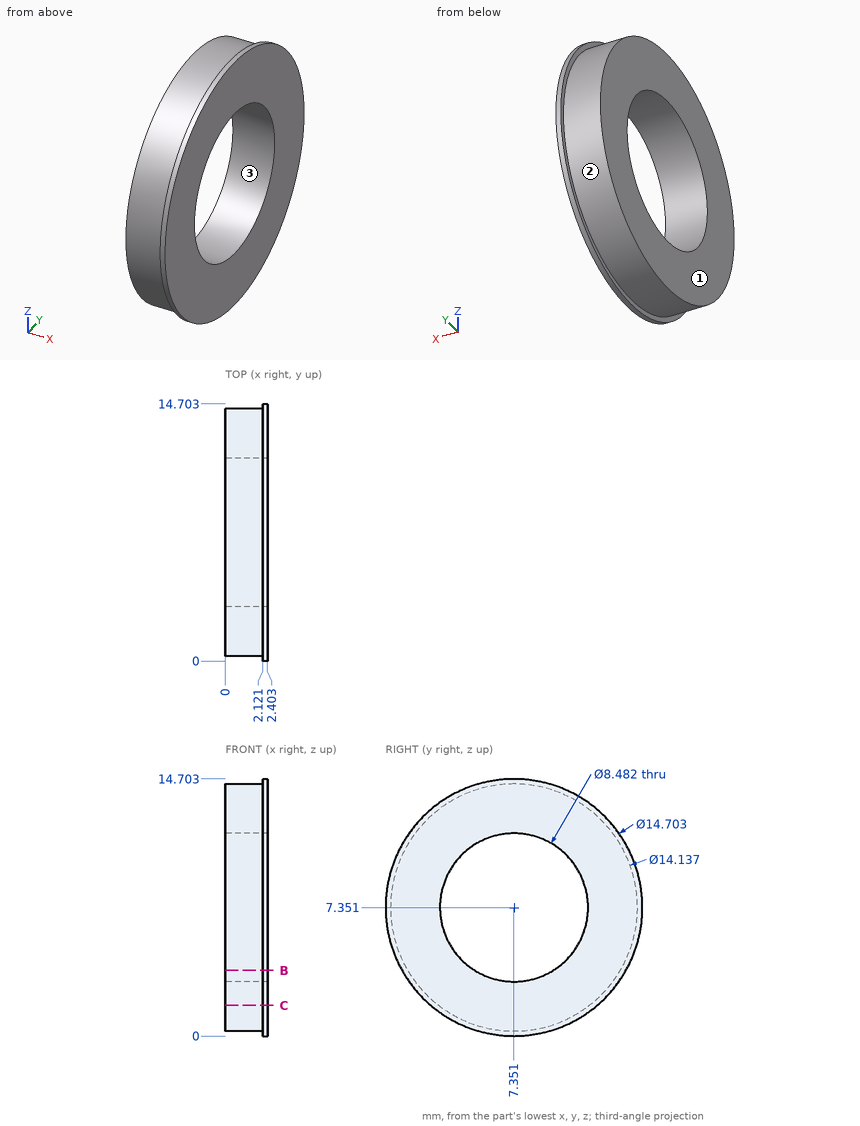
Input: dimensioned drawing with shaded views. Units: mm. Origin: part minimum x, y, z. Round coordinates to 2 decimals unless told otherwise and drop trailing zeros. Loops run counter-clockwise (first coordinate to the right, second up) from the corner with the lowest first, then second, coordinate; pieces in that order, holes last. Notation, with made-up numbers: (77, -20) -> (82, -20) arc R32 ccw to (82, 12) -> close; hole circle Ø11 at (-22.75, 70.25). An arc over 180 degrees is marked (long way). Answer as a JSON object with one key per item and string values. Group by question number.
1) Ray query, L1, parallel to Y at x = 2, z = 7.25; L2, parallel to Y at x = 1.5, z = 4.5 (1 decimal); L3, parallel to Z at x = 1.1, y = 4.25 (1 decimal). Return the intervals inside material, ascending.
2) Pin query (flat end, axial travel): pin 1 (7 mm diameter, centred on y = 7.35, z = 7.35, fed in from -X). Return the tip coordinate at first contact, or that it passes through.
3) Section query C-C on z = 1.75. Output: boundary loops of the cut face in (x, y), plus the area to 3 significant figures.
4) Section query B-B on z = 3.75. Output: boundary loops of the cut face in (x, y).
5) Draft query along Z for the marked faces 1, 2 and 3. Return one class per face: +Z half, -Z half, draft (parallel to the pull), parting line (faces both ways), or undercut.
Reply:
{
 "1": {"L1": "y = 0.28 to 3.11, 11.59 to 14.42", "L2": "y = 0.9 to 4.2, 10.5 to 13.8", "L3": "z = 1 to 4.5, 10.2 to 13.7"},
 "2": {"pin 1": "passes through"},
 "3": {"outline": "(0, 3.04) -> (2.12, 3.04) -> (2.12, 2.59) -> (2.4, 2.59) -> (2.4, 12.11) -> (2.12, 12.11) -> (2.12, 11.66) -> (0, 11.66) -> close", "area": "21.0 mm2"},
 "4": {"outline": "(0, 1.27) -> (2.12, 1.27) -> (2.12, 0.94) -> (2.4, 0.94) -> (2.4, 5.11) -> (0, 5.11) -> close; (0, 9.59) -> (2.4, 9.59) -> (2.4, 13.76) -> (2.12, 13.76) -> (2.12, 13.43) -> (0, 13.43) -> close"},
 "5": {"face 1": "draft", "face 2": "parting line", "face 3": "undercut"}
}
